from build123d import *

# Parameters (mm, degrees)
BOSS_EXTRUDE1_DEPTH = 3.175
SKETCH1_3_W         = 76.2
SKETCH1_3_H         = 6.843416336
BOSS_EXTRUDE2_DEPTH = 3.175
FILLET1_R           = 0.762


with BuildPart() as part:
    # Sketch1 → Boss-Extrude1 (new body)
    with BuildSketch(Plane(origin=(0, 0, 0), x_dir=(0, 0, -1), z_dir=(1, 0, 0))):
        with BuildLine():
            Line((-43.663217685, -8.64329225), (-43.663217685, -11.81829225))
            Line((-43.663217685, -11.81829225), (-38.1, -11.81829225))
            Line((-38.1, -11.81829225), (38.1, -11.81829225))
            Line((38.1, -11.81829225), (43.663218279, -11.81829225))
            Line((43.663218279, -11.81829225), (43.663218279, -8.64329225))
            Line((43.663218279, -8.64329225), (53.425755965, -8.64329225))
            add(Edge.make_bspline(
                [(53.425755965, -8.64329225), (53.263215222, -8.501846261), (52.438865838, -7.790883032), (51.598732776, -7.098646879), (50.924889325, -6.543426735)],
                knots=[0.589295503, 0.589295503, 0.589295503, 0.589295503, 0.670587257, 1, 1, 1, 1], degree=3))
            add(Edge.make_bspline(
                [(50.924889325, -6.543426735), (50.124144808, -5.909206331), (48.528125823, -4.645098009), (46.059087128, -2.864191401), (43.549887667, -1.177645044), (40.997889023, 0.406107926), (38.408155063, 1.888342774), (35.783665586, 3.267940071), (33.127912186, 4.544590036), (30.444209343, 5.717936201), (27.735877167, 6.787796608), (25.006192871, 7.754099696), (22.258403703, 8.616894329), (19.495723603, 9.376346971), (16.721334228, 10.032717883), (13.938384845, 10.586434135), (11.149992554, 11.03779968), (8.359242424, 11.388052771), (5.569187679, 11.635427625), (2.782849792, 11.78974762), (0.926482231, 11.808788455), (1.344e-06, 11.818291406)],
                knots=[0, 0, 0, 0, 0.055514859, 0.110650485, 0.165414313, 0.219814889, 0.273861748, 0.327565289, 0.380936647, 0.43398757, 0.486730286, 0.53917738, 0.59134167, 0.643236089, 0.694873565, 0.746266915, 0.797428738, 0.848371322, 0.899106551, 0.949645827, 1, 1, 1, 1], degree=3))
            add(Edge.make_bspline(
                [(1.344e-06, 11.818291406), (-0.978048688, 11.807700808), (-2.937955589, 11.78647839), (-5.879617768, 11.614460814), (-8.825050086, 11.338662737), (-11.770693383, 10.948099308), (-14.712949005, 10.444720364), (-17.648178684, 9.827137854), (-20.57270433, 9.095020044), (-23.482807764, 8.247912067), (-26.374730804, 7.285560858), (-29.244674098, 6.207832855), (-32.088800801, 5.014747428), (-34.903222204, 3.706458544), (-37.684051606, 2.283328938), (-40.427201271, 0.74568464), (-43.129148213, -0.90523213), (-45.784047279, -2.670825623), (-48.3946206, -4.541678592), (-50.079432356, -5.874568434), (-50.924883817, -6.543422779)],
                knots=[0, 0, 0, 0, 0.053156962, 0.106520825, 0.160104405, 0.213921194, 0.267985268, 0.32231118, 0.376913837, 0.431808373, 0.48701001, 0.542533909, 0.598395017, 0.654607907, 0.711186615, 0.76814447, 0.825493932, 0.883246422, 0.941412159, 1, 1, 1, 1], degree=3))
            add(Edge.make_bspline(
                [(-50.924883817, -6.543422779), (-51.598727834, -7.098643313), (-52.438862565, -7.790880746), (-53.263213559, -8.501845329), (-53.425755371, -8.64329225)],
                knots=[0, 0, 0, 0, 0.32941274, 0.410704965, 0.410704965, 0.410704965, 0.410704965], degree=3))
            Line((-53.425755371, -8.64329225), (-43.663217685, -8.64329225))
        make_face()
    extrude(amount=-BOSS_EXTRUDE1_DEPTH)

    # Sketch1<3> → Boss-Extrude2 (add)
    with BuildSketch(Plane(origin=(0, 0, 0), x_dir=(0, 0, -1), z_dir=(1, 0, 0))):
        with Locations((0, -15.240000418)):
            Rectangle(SKETCH1_3_W, SKETCH1_3_H)
    extrude(amount=-BOSS_EXTRUDE2_DEPTH)

    # Fillet1
    fillet1_edges = [part.edges().sort_by_distance(p)[0] for p in [
        (-1.5875, -8.64329225, -53.425755965),
        (-1.5875, -8.64329225, -43.663218279),
        (-1.5875, -11.81829225, -43.663218279),
        (-1.5875, -11.81829225, 43.663217685),
        (-1.5875, -8.64329225, 43.663217685),
        (-1.5875, -8.64329225, 53.425755371),
        (-1.5875, -18.661708586, -38.1),
        (-1.5875, -11.81829225, -38.1),
        (-1.5875, -18.661708586, 38.1),
        (-1.5875, -11.81829225, 38.1),
    ]]
    fillet(fillet1_edges, radius=FILLET1_R)


solid = part.part
Part model, mm, in its own coordinate system. A direction names the side the tool comes from. Give positions to 0.01 mm unless a question says otherwise; leave off trailing zeros. Loops run counter-clockwise (first coordinate to the right, second up) from the corner with the lowest first, then second, coordinate; pieces in that order, holes last. Notation, with made-up numbers: M 64,-18 L 82,-18 A20 ccw 82,-4 Z; hole C 0.25,-20 d5. An arc over 180 degrees is marked long. Put each result on its own line as item: value. Start each with the question number.
1) Probe probe 1 along Z at (x, y) = (-0.2, -16); probe 2 along Z at (x, y) = (-2, -10.5); probe 3 along Y at (x, z) = (-1.35, -16). List the from-to ranges inside material, lowest first.
2) Saw through at A-A (y = -15). List the corners of the cut face in (x, z) (3 decimals).
3) 3-axis set-ups, long thin cutter, end or side, ignore diameter. For faces 1 (the flat face through (-3.175, -3, 1)), 2 (the flat face through (-2, -10, -43.663)), 3 (the flat face through (-2, -15, 38.1)): which of +Z, -Z, +X, -X, +Y, -Y reach the whole face in a straight line?
4) Flat gauge pins, fed straight in: pin 1 (1.8 mm diameter, centred on x = -2, y = -10.5, fed in from -Z); pin 2 (1.6 mm diameter, centred on x = -2.5, z = 49, fed in from -Y); pin 3 (1 mm diameter, centred on x = -1.5, y = -15, fed in from +Z). Where does each tip first touch, or does it go through?
Numbers:
1. probe 1: -38.1 to 38.1
1. probe 2: -43.66 to 43.66
1. probe 3: -18.66 to 10.17
2. outline: M -3.175,-38.1 L 0,-38.1 L 0,38.1 L -3.175,38.1 Z
3. face 1: +Z, -Z, -X, +Y, -Y
3. face 2: -Z, +X, -X, -Y
3. face 3: +Z, +X, -X, -Y
4. pin 1: z = -43.66
4. pin 2: y = -8.64
4. pin 3: z = 38.1
